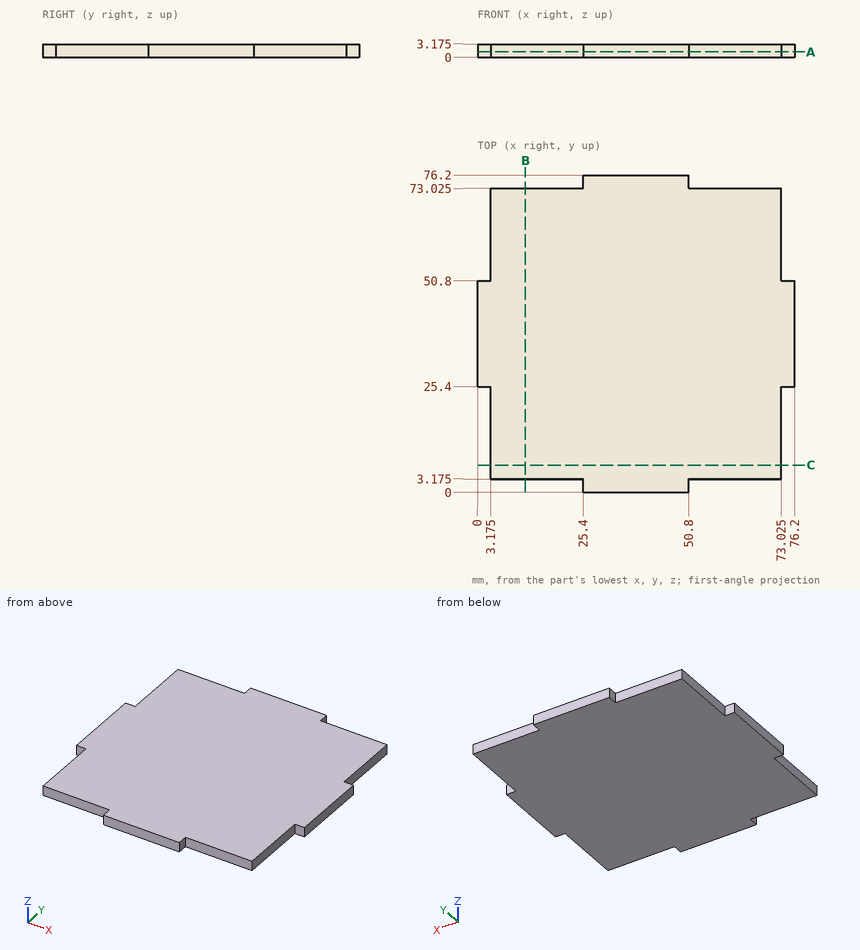
Part print with two shaded views. Sizes in mm from the minimum x, y, z corner. Coordinates: 2 decimals unless noted, no trailing zeros. Write each loop counter-clockwise with the first axis right and the second up, starting at its lowest first coordinate (ties: lowest second). Pieces come first, ordered by that corner, then holes. Notation, with made-up numbers: (-33.75, -9) -> (-9.75, -9) arc R13 cw to (-9.75, 13) -> close; hole circle Ø9 at (39.5, -17.75). An arc over 180 degrees is marked (long way). Return JSON: item names as keys, results as strings. Group by question number.
Q1. Flat gauge pins, fed straight in: pin 1 (1 mm diameter, centred on y = 58.5, z = 2, fed in from -X) (3 decimals); pin 2 (1 mm diameter, centred on y = 62.5, z = 2.5, fed in from +X) (3 decimals); pin 3 (1 mm diameter, centred on y = 74.5, z = 1, fed in from -X). Where does each tip first touch, or does it go through?
Q2. Cut at B-B, the plane x = 11.5. Give the cut face in (y, z) (3 decimals), then the cut area to 3 significant figures.
Q3. Drill centre lines: line 1 (X direction, y = 72.5, z = 2.3) (3 decimals); line 2 (Y direction, x = 73.5, z = 0.95). Where is each one in solid material? Low to high.
Q4. Cut at A-A, the plane z = 1.3. Give the cut face in (x, y) (3 decimals), then the cut area to 3 significant figures.
Returned:
{
 "1": {"pin 1": "stops at x = 3.175", "pin 2": "stops at x = 73.025", "pin 3": "stops at x = 25.4"},
 "2": {"outline": "(3.175, 0) -> (73.025, 0) -> (73.025, 3.175) -> (3.175, 3.175) -> close", "area": "222 mm2"},
 "3": {"line 1": "x = 3.175 to 73.025", "line 2": "y = 25.4 to 50.8"},
 "4": {"outline": "(0, 25.4) -> (3.175, 25.4) -> (3.175, 3.175) -> (25.4, 3.175) -> (25.4, 0) -> (50.8, 0) -> (50.8, 3.175) -> (73.025, 3.175) -> (73.025, 25.4) -> (76.2, 25.4) -> (76.2, 50.8) -> (73.025, 50.8) -> (73.025, 73.025) -> (50.8, 73.025) -> (50.8, 76.2) -> (25.4, 76.2) -> (25.4, 73.025) -> (3.175, 73.025) -> (3.175, 50.8) -> (0, 50.8) -> close", "area": "5,200 mm2"}
}
